Read the model definition and answer for the solid it produces. Units are mm, in the model's axes. Face numbers are marked on the shaded views. A direction names the side the tool comes from. Give positions to 0.01 mm unless a question says otherwise; leave off trailing zeros. Loops run counter-clockwise (first coordinate to the right, second up) from the corner with the lowest first, then second, coordinate; pieces in that order, holes last. Notation, with made-up numbers: M 71.25,-17 L 125.25,-17 A27 ccw 125.25,17 Z; hole C 82.25,26.5 d9. An arc over 180 degrees is marked long. Return JSON: item names as keys, results as strings. Group by question number.
```python
from build123d import *

# Parameters (mm, degrees)
BOSS_EXTRUDE1_DEPTH = 6.35
BOSS_EXTRUDE2_DEPTH = 101.6
FILLET1_R           = 12.7
FILLET2_R           = 12.7


with BuildPart() as part:
    # Sketch1 → Boss-Extrude1 (new body)
    # profile 1 of 2: a face of its own
    with BuildSketch(Plane(origin=(0, 0, 0), x_dir=(1, 0, 0), z_dir=(0, 1, 0))):
        Polygon((127, -141.108591334), (127, 141.108591334), (77.608591334, 190.5), (-77.608591334, 190.5), (-127, 141.108591334), (-127, -141.108591334), (-77.608591334, -190.5), (77.608591334, -190.5), align=None)
        Polygon((-120.65, -138.478335213), (-120.65, 138.478335213), (-74.978335213, 184.15), (74.978335213, 184.15), (120.65, 138.478335213), (120.65, -138.478335213), (74.978335213, -184.15), (-74.978335213, -184.15), align=None, mode=Mode.SUBTRACT)
    # profile 2 of 2: a face of its own
    with BuildSketch(Plane(origin=(0, 0, 0), x_dir=(1, 0, 0), z_dir=(0, 1, 0))):
        Polygon((-120.65, 138.478335213), (-74.978335213, 184.15), (74.978335213, 184.15), (120.65, 138.478335213), (120.65, -138.478335213), (74.978335213, -184.15), (-74.978335213, -184.15), (-120.65, -138.478335213), align=None)
        with BuildLine():
            ThreePointArc((-31.75, -63.5), (0, -95.25), (31.75, -63.5))
            Line((31.75, -63.5), (31.75, 63.5))
            ThreePointArc((31.75, 63.5), (0, 95.25), (-31.75, 63.5))
            Line((-31.75, 63.5), (-31.75, -63.5))
        make_face(mode=Mode.SUBTRACT)
    extrude(amount=BOSS_EXTRUDE1_DEPTH)

    # Sketch1_4 → Boss-Extrude2 (add)
    with BuildSketch(Plane(origin=(0, 0, 0), x_dir=(1, 0, 0), z_dir=(0, 1, 0))):
        Polygon((127, -141.108591334), (127, 141.108591334), (77.608591334, 190.5), (-77.608591334, 190.5), (-127, 141.108591334), (-127, -141.108591334), (-77.608591334, -190.5), (77.608591334, -190.5), align=None)
        Polygon((-120.65, -138.478335213), (-120.65, 138.478335213), (-74.978335213, 184.15), (74.978335213, 184.15), (120.65, 138.478335213), (120.65, -138.478335213), (74.978335213, -184.15), (-74.978335213, -184.15), align=None, mode=Mode.SUBTRACT)
    extrude(amount=BOSS_EXTRUDE2_DEPTH)

    # Fillet1
    fillet1_edges = [part.edges().sort_by_distance(p)[0] for p in [
        (127, 50.8, 141.108591334),
        (77.608591334, 50.8, 190.5),
        (-77.608591334, 50.8, 190.5),
        (-127, 50.8, 141.108591334),
        (-127, 50.8, -141.108591334),
        (-77.608591334, 50.8, -190.5),
        (77.608591334, 50.8, -190.5),
        (127, 50.8, -141.108591334),
    ]]
    fillet(fillet1_edges, radius=FILLET1_R)

    # Fillet2
    fillet2_edges = [part.edges().sort_by_distance(p)[0] for p in [
        (-120.65, 53.975, 138.478335213),
        (-120.65, 53.975, -138.478335213),
        (-74.978335213, 53.975, -184.15),
        (74.978335213, 53.975, -184.15),
        (120.65, 53.975, -138.478335213),
        (120.65, 53.975, 138.478335213),
        (74.978335213, 53.975, 184.15),
        (-74.978335213, 53.975, 184.15),
    ]]
    fillet(fillet2_edges, radius=FILLET2_R)


solid = part.part
```
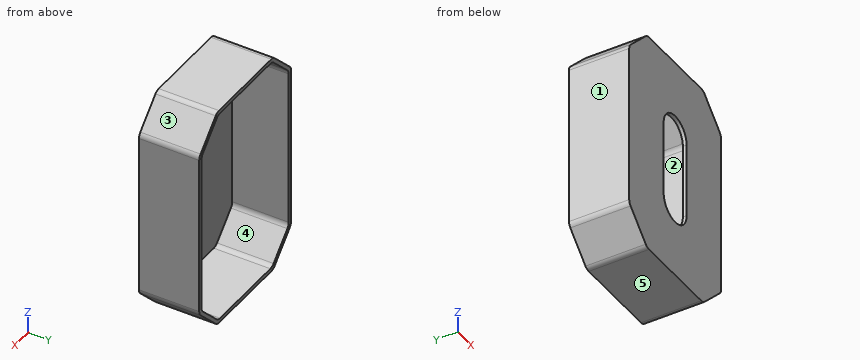
1. Straight lines are drawn through the part: line 1 along X through (y, z) = (46.5, -6); line 2 along Z through (x, y) = (62, 11); line 3 along Y through (x, z) = (71.5, 112.5). For each, find the intervals that lie inside material, in ascending order.
2. Find section A-A (z = 19.5). Write down the section's boundary in (x, y).
3. Flat-ended cylindrical pins translate along their axes: P1, Ø4, axis at x = 10, z = -139, coming from the +Y side; P2, Ø4, axis at x = 80.5, y = 38.5, coming from the -Z side. Find the tip coordinate at first contact, or state that the pin passes through.
4. Find section B-B (x = 0). Write down the section's boundary in (y, z).
5. For the marked faces 4 and 5, determine the directions among +Z, -Z, +X, -X, +Y, -Y from which every point of the face is accessible in a straight line to the end or side of a thin tool.
6. The mould has two halves that part along X. Classify the marked faces 1, 2 and 3: +X half, -X half, draft (parallel to the pull), parting line (faces both ways), or undercut.
7. Find section D-D (z = -110). Write down the section's boundary in (x, y).
Result:
{
 "1": {"line 1": "x = -127 to -120.65, 120.65 to 127", "line 2": "z = -190.5 to -184.15, 184.15 to 190.5", "line 3": "y = 0 to 6.35"},
 "2": {"outline": "M -127,0 L -31.75,0 L -31.75,6.35 L -120.65,6.35 L -120.65,101.6 L -127,101.6 Z; M 31.75,0 L 127,0 L 127,101.6 L 120.65,101.6 L 120.65,6.35 L 31.75,6.35 Z"},
 "3": {"P1": "stops at y = 6.35", "P2": "stops at z = -188.91"},
 "4": {"outline": "M 0,-190.5 L 101.6,-190.5 L 101.6,-184.15 L 6.35,-184.15 L 6.35,-95.25 L 0,-95.25 Z; M 0,95.25 L 6.35,95.25 L 6.35,184.15 L 101.6,184.15 L 101.6,190.5 L 0,190.5 Z"},
 "5": {"face 4": "+Y", "face 5": "-Z, +X, -X, +Y, -Y"},
 "6": {"face 1": "-X half", "face 2": "undercut", "face 3": "+X half"},
 "7": {"outline": "M -127,0 L 127,0 L 127,101.6 L 120.65,101.6 L 120.65,6.35 L -120.65,6.35 L -120.65,101.6 L -127,101.6 Z"}
}
